Geometry check sheet. Reference: the model listing, model coordinates, mm. A direction names the side the tool comes from. Round coordinates to 2 decimals unless told otherwise and drop trailing zeros. Order: outer loops, then holes, each group sorted by start corner. A loop starts at its lowest first (then second) coordinate and runs counter-clockwise, first axis right, second up.
(1) Thickness scan on L1, parallel to Z at x = 4.5, y = 13.6; L2, parallel to X at y = 13.55, z = 2.5; L3, parallel to Z at x = 14.5, y = 5. Record the ranges inside material, lowest first.
(2) Gauge pin test, flat ends, axial feed: P1, Ø2, axis at y = 14, z = 2, coming from the +X side; P2, Ø0.7, axis at y = 5.5, z = 3, coming from the +X side. Record the tip position at first contact, or that the pin passes through.
(3) Cross-section at B-B on y = 10.5. Enter the section's corners in (x, z).
(4) Set-up check for faces 1 (the face through (1, 2.5, 17)), 2 (the face through (4.5, 12.5, 17.4)), 3 (the face through (13.69, 2.021, 16.345)), 4 (the face through (14, 4.9, 3)): record each of +Z, -Z, +X, -X, +Y, -Y from which the full face is reachable in a straight line by a thin tool's end or side.
(5) Cross-section at C-C on y = 6.25. Enter the section's corners in (x, z), and give its area (3 significant figures).
(6) Draft check along Z on faces 5 (the face through (13, 5.5, 10)), 6 (the face through (13.7, 0, 2.4)). Enter one of: pulls with the +Z half, pulls with the -Z half, needs draft (parallel to the pull), parting line crosses it, or undercut.
(7) Cross-section at A-A on x = 14. Enter the section's corners in (y, z), and give its area (3 significant figures).
from build123d import *

# Parameters (mm, degrees)
EXTRUDE_1_DEPTH        = 25
SKETCH_2_R             = 1.25
EXTRUDE_2_DEPTH        = 8.5
PATTERN_LINEAR_1_COUNT = 5
PATTERN_LINEAR_1_PITCH = 5
SKETCH_3_W             = 3
SKETCH_3_H             = 3.3
CUT_EXTRUDE_1_DEPTH    = 3
PATTERN_LINEAR_2_COUNT = 5
PATTERN_LINEAR_2_PITCH = 5
CUT_EXTRUDE_2_DEPTH    = 0.1
SKETCH_5_W             = 25
SKETCH_5_H             = 1
CUT_EXTRUDE_3_DEPTH    = 0.1
SKETCH_6_R             = 1.9
CUT_EXTRUDE_4_DEPTH    = 2
PATTERN_LINEAR_3_COUNT = 5
PATTERN_LINEAR_3_PITCH = 5
SKETCH_7_W             = 1
SKETCH_7_H             = 3
CUT_EXTRUDE_5_DEPTH    = 2
PATTERN_LINEAR_4_COUNT = 5
PATTERN_LINEAR_4_PITCH = 5
CUT_EXTRUDE_6_DEPTH    = 0.5
PATTERN_LINEAR_5_COUNT = 5
PATTERN_LINEAR_5_PITCH = 5
SKETCH_9_W             = 18
SKETCH_9_H             = 15
CUT_EXTRUDE_7_DEPTH    = 5


with BuildPart() as part:
    # Эскиз1 → Вытянуть1 (new body)
    with BuildSketch(Plane.XY):
        Polygon((0, 0), (9.5, 0), (9.5, 5.5), (8.5, 5.5), (8.5, 15), (0, 15), align=None)
    extrude(amount=EXTRUDE_1_DEPTH)

    # Эскиз2 → Вытянуть2 (add)
    with BuildSketch(Plane(origin=(9.5, 0, 0), x_dir=(0, 0, -1), z_dir=(1, 0, 0))):
        with BuildLine():
            Line((-25, 5.5), (-24, 5.5))
            Line((-24, 5.5), (-24, 4.9))
            Line((-24, 4.9), (-21, 4.9))
            Line((-21, 4.9), (-21, 5.5))
            Line((-21, 5.5), (-20, 5.5))
            Line((-20, 5.5), (-20, 2.5))
            ThreePointArc((-20, 2.5), (-22.5, 0), (-25, 2.5))
            Line((-25, 2.5), (-25, 5.5))
        make_face()
        with Locations((-22.5, 2.5)):
            Circle(SKETCH_2_R, mode=Mode.SUBTRACT)
    extrude_2 = extrude(amount=EXTRUDE_2_DEPTH)

    # Линейный массив1: Вытянуть2 ×5
    with Locations(*[(0, 0, -i * PATTERN_LINEAR_1_PITCH) for i in range(1, PATTERN_LINEAR_1_COUNT)]):
        add(extrude_2)

    # Эскиз3 → Вырез-Вытянуть1 (cut)
    with BuildSketch(Plane.ZY):
        with Locations((2.5, 4.15)):
            Rectangle(SKETCH_3_W, SKETCH_3_H)
    cut_extrude_1 = extrude(amount=-CUT_EXTRUDE_1_DEPTH, mode=Mode.SUBTRACT)

    # Линейный массив2: Вырез-Вытянуть1 ×5
    with Locations(*[(0, 0, i * PATTERN_LINEAR_2_PITCH) for i in range(1, PATTERN_LINEAR_2_COUNT)]):
        add(cut_extrude_1, mode=Mode.SUBTRACT)

    # Эскиз4 → Вырез-Вытянуть2 (cut)
    with BuildSketch(Plane.ZY):
        Polygon((0, 13.5), (25, 13.5), (25, 12.5), (25.5, 12.5), (25.5, 7), (24.5, 7), (24.5, 12.5), (20.5, 12.5), (20.5, 7), (19.5, 7), (19.5, 12.5), (15.5, 12.5), (15.5, 7), (14.5, 7), (14.5, 12.5), (10.5, 12.5), (10.5, 7), (9.5, 7), (9.5, 12.5), (5.5, 12.5), (5.5, 7), (4.5, 7), (4.5, 12.5), (0, 12.5), align=None)
    extrude(amount=-CUT_EXTRUDE_2_DEPTH, mode=Mode.SUBTRACT)

    # Эскиз5 → Вырез-Вытянуть3 (cut)
    with BuildSketch(Plane.ZY):
        with Locations((12.5, 1)):
            Rectangle(SKETCH_5_W, SKETCH_5_H)
    extrude(amount=-CUT_EXTRUDE_3_DEPTH, mode=Mode.SUBTRACT)

    # Эскиз6 → Вырез-Вытянуть4 (cut)
    with BuildSketch(Plane(origin=(0, 15, 0), x_dir=(-1, 0, 0), z_dir=(0, 1, 0))):
        with Locations(Location((-4.5, 2.5, 0), (0, 0, 90))):
            Circle(SKETCH_6_R)
    cut_extrude_4 = extrude(amount=-CUT_EXTRUDE_4_DEPTH, mode=Mode.SUBTRACT)

    # Линейный массив3: Вырез-Вытянуть4 ×5
    with Locations(*[(0, 0, i * PATTERN_LINEAR_3_PITCH) for i in range(1, PATTERN_LINEAR_3_COUNT)]):
        add(cut_extrude_4, mode=Mode.SUBTRACT)

    # Эскиз7 → Вырез-Вытянуть5 (cut)
    with BuildSketch(Plane(origin=(0, 15, 0), x_dir=(-1, 0, 0), z_dir=(0, 1, 0))):
        with Locations((-1.5, 2.5)):
            Rectangle(SKETCH_7_W, SKETCH_7_H)
    cut_extrude_5 = extrude(amount=-CUT_EXTRUDE_5_DEPTH, mode=Mode.SUBTRACT)

    # Линейный массив4: Вырез-Вытянуть5 ×5
    with Locations(*[(0, 0, i * PATTERN_LINEAR_4_PITCH) for i in range(1, PATTERN_LINEAR_4_COUNT)]):
        add(cut_extrude_5, mode=Mode.SUBTRACT)

    # Эскиз8 → Вырез-Вытянуть6 (cut)
    with BuildSketch(Plane(origin=(0, 13, 0), x_dir=(-1, 0, 0), z_dir=(0, 1, 0))):
        Polygon((-6.185425231, 3.377121309), (-3.325012579, 1.006880929), (-2.814574769, 1.622878691), (-5.674987421, 3.993119071), align=None)
    cut_extrude_6 = extrude(amount=-CUT_EXTRUDE_6_DEPTH, mode=Mode.SUBTRACT)

    # Линейный массив5: Вырез-Вытянуть6 ×5
    with Locations(*[(0, 0, i * PATTERN_LINEAR_5_PITCH) for i in range(1, PATTERN_LINEAR_5_COUNT)]):
        add(cut_extrude_6, mode=Mode.SUBTRACT)

    # Эскиз9 → Вырез-Вытянуть7 (cut)
    with BuildSketch(Plane.XY.offset(25)):
        with Locations((9, 7.5)):
            Rectangle(SKETCH_9_W, SKETCH_9_H)
    extrude(amount=-CUT_EXTRUDE_7_DEPTH, mode=Mode.SUBTRACT)


solid = part.part
Found:
1. L1: z = 0 to 0.6, 4.4 to 5.6, 9.4 to 10.6, 14.4 to 15.6, 19.4 to 20
1. L2: x = 0 to 1, 2 to 2.6, 6.4 to 8.5
1. L3: z = 0 to 1, 4 to 6, 9 to 11, 14 to 16, 19 to 20
2. P1: stops at x = 8.5
2. P2: stops at x = 9.5
3. outline: (0, 0) - (8.5, 0) - (8.5, 20) - (0.1, 20) - (0.1, 19.5) - (0, 19.5) - (0, 15.5) - (0.1, 15.5) - (0.1, 14.5) - (0, 14.5) - (0, 10.5) - (0.1, 10.5) - (0.1, 9.5) - (0, 9.5) - (0, 5.5) - (0.1, 5.5) - (0.1, 4.5) - (0, 4.5) - close
4. face 1: -X
4. face 2: +Y
4. face 3: +X
4. face 4: +X, +Y
5. outline: (0, 0) - (8.5, 0) - (8.5, 20) - (0, 20) - close
5. area: 170 mm2
6. face 5: needs draft
6. face 6: undercut
7. outline: (2.5, 0) - (5.5, 0) - (5.5, 1) - (4.9, 1) - (4.9, 4) - (5.5, 4) - (5.5, 6) - (4.9, 6) - (4.9, 9) - (5.5, 9) - (5.5, 11) - (4.9, 11) - (4.9, 14) - (5.5, 14) - (5.5, 16) - (4.9, 16) - (4.9, 19) - (5.5, 19) - (5.5, 20) - (2.5, 20) arc R2.5 ccw to (2.5, 15) arc R2.5 ccw to (2.5, 10) arc R2.5 ccw to (2.5, 5) arc R2.5 ccw to start; hole circle Ø2.5 at (2.5, 2.5); hole circle Ø2.5 at (2.5, 7.5); hole circle Ø2.5 at (2.5, 12.5); hole circle Ø2.5 at (2.5, 17.5)
7. area: 72.4 mm2
